CAD build for the part. Positions are in the model's coordinates, mm. Give positions to 0.01 mm unless a question says otherwise; leave off trailing zeros. Order: outer loops, then holes, each group sorted by start corner. A loop starts at its lowest first (then second) coordinate and runs counter-clockwise, first axis right, second up. Notation, with made-up numbers: (26.5, 49.25) -> (56.5, 49.25) arc R25 cw to (56.5, 72.25) -> close; hole circle Ø1 at (4.5, -38). An arc over 180 degrees is marked (long way). Use one line per item in the form item = value. Start each with the question number.
1) Drop a flat-ended pin along its axis: P1, Ø5, axis at x = 63.5, y = -44.45, coming from the -Z side. Give the stop position or say it passes through.
2) Cut at D-D, the plane y = -12.7. Give the cut face in (x, z) (3 decimals), and give its area (3 significant figures).
3) Cut at A-A, the plane y = -44.45. Give the cut face in (x, z) (3 decimals).
4) Cut at C-C, the plane x = 12.7. Give the cut face in (y, z) (1 decimal), and give its area (3 significant figures).
5) Probe line 1 (Y direction, x = 63.5, z = 0.65) (3 decimals); line 2 (X direction, y = -13, z = 2.95); line 3 (X direction, y = -15.5, z = 2.6). List the from-to ranges inside material, lowest first.
6) Cut at B-B, the plane z = 1.9. State how many separate pieces and enclosed holes the cut face has, and give its area (3 significant figures).
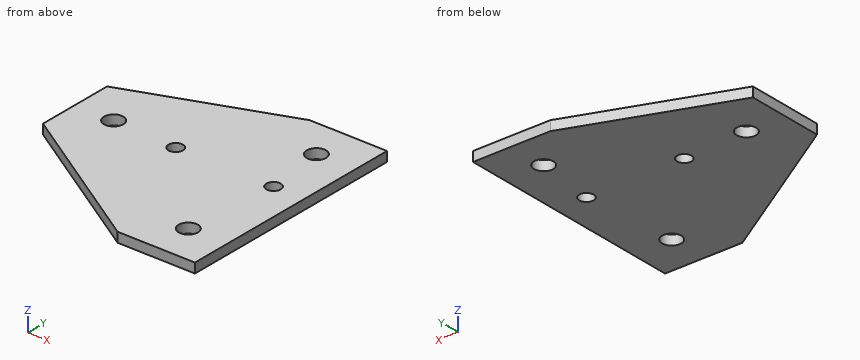
Autodesk Inventor part; units mm, degrees
ref_plane "YZ Plane" through (0, 0, 0) normal (1, 0, 0) x (0, 1, 0)
ref_plane "XZ Plane" through (0, 0, 0) normal (0, 1, 0) x (-1, 0, 0)
ref_plane "XY Plane" through (0, 0, 0) normal (0, 0, 1) x (1, 0, 0)
sketch "Sketch1" plane through (0, 0, 0) normal (0, 0, 1) x (1, 0, 0)
  line L0 (0, 0) -> (50.8, 19.05)
  line L1 (50.8, 19.05) -> (76.2, 19.05)
  line L2 (76.2, 19.05) -> (76.2, -57.15)
  line L3 (76.2, -57.15) -> (50.8, -57.15)
  line L4 (50.8, -57.15) -> (0, -25.4)
  line L5 (0, -25.4) -> (0, 0)
  line L6 (76.2, -6.35) -> (26.8732, -6.35) construction
  line L7 (26.8732, -6.35) -> (26.8732, -41.7576) construction
  line L8 (26.8732, -41.7576) -> (76.2, -41.7576) construction
  line L9 (76.2, -41.7576) -> (76.2, -6.35) construction
  circle A0 centre (33.8732, -13.65) radius 2.3813
  circle A1 centre (66.0064, -13.65) radius 2.3813
  line L10 (0, 0) -> (76.2, 0) construction
  circle A2 centre (12.7, -12.7) radius 3.175
  circle A3 centre (63.5, -44.45) radius 3.175
  circle A4 centre (63.5, 6.35) radius 3.175
  dimension "d0" = 25.4
  dimension "d1" = 76.2
  dimension "d2" = 19.05
  dimension "d3" = 76.2
  dimension "d4" = 25.4
  dimension "d5" = 25.4
  dimension "d6" = 49.3268
  dimension "d7" = 35.4076
  dimension "d8" = 25.4
  dimension "d10" = 7.3
  dimension "d11" = 7.3
  dimension "d15" = 10.1936
  dimension "d16" = 7
  dimension "d18" = 6.35
  dimension "d19" = 12.7
  dimension "d20" = 12.7
  dimension "d21" = 6.35
  dimension "d22" = 6.35
  dimension "d23" = 12.7
  dimension "d24" = 12.7
  dimension "d25" = 12.7
  dimension "d26" = 12.7
  dimension "d29" = 4.7625
extrude "Extrusion1" add sketch "Sketch1" along normal blind 3.175
properties part number "15102898-16-P-0309_CPY1" material "Aluminum 6061"
Result:
q1.P1 = through
q2.outline = (0, 0) -> (9.525, 0) -> (9.525, 3.175) -> (0, 3.175) -> close; (15.875, 0) -> (31.69, 0) -> (31.69, 3.175) -> (15.875, 3.175) -> close; (36.057, 0) -> (63.823, 0) -> (63.823, 3.175) -> (36.057, 3.175) -> close; (68.19, 0) -> (76.2, 0) -> (76.2, 3.175) -> (68.19, 3.175) -> close
q2.area = 194 mm²
q3.outline = (30.48, 0) -> (60.325, 0) -> (60.325, 3.175) -> (30.48, 3.175) -> close; (66.675, 0) -> (76.2, 0) -> (76.2, 3.175) -> (66.675, 3.175) -> close
q4.outline = (-33.3, 0) -> (-15.9, 0) -> (-15.9, 3.2) -> (-33.3, 3.2) -> close; (-9.5, 0) -> (4.8, 0) -> (4.8, 3.2) -> (-9.5, 3.2) -> close
q4.area = 101 mm²
q5.line_1 = -57.15 to -47.625, -41.275 to 3.175, 9.525 to 19.05
q5.line_2 = 0 to 9.54, 15.86 to 31.58, 36.16 to 63.72, 68.3 to 76.2
q5.line_3 = 0 to 11.2, 14.2 to 32.37, 35.37 to 64.51, 67.51 to 76.2
q6.separate_pieces = 1
q6.enclosed_holes = 5
q6.area = 4,390 mm²
